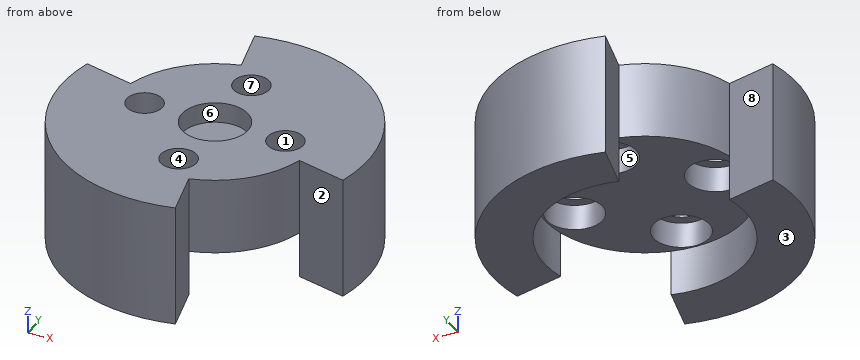
```python
from build123d import *

# Parameters (mm, degrees)
SKETCH012_R     = 9.9
SKETCH012_R_2   = 1.75
PAD009_DEPTH    = 5
SKETCH013_R     = 9.9
SKETCH013_R_2   = 2.75
PAD010_DEPTH    = 2.5
SKETCH014_R     = 3.25
POCKET002_DEPTH = 2
PAD011_DEPTH    = 12


with BuildPart() as part:
    # Sketch012 (on DatumPlane) → Pad009 (new body)
    with BuildSketch(Plane(origin=(0, 0, -19.5), x_dir=(-1, 0, 0), z_dir=(0, 0, -1))):
        Circle(SKETCH012_R)
        with Locations((0, 7)):
            Circle(SKETCH012_R_2, mode=Mode.SUBTRACT)
        with Locations((7, 0)):
            Circle(SKETCH012_R_2, mode=Mode.SUBTRACT)
        with Locations((0, -7)):
            Circle(SKETCH012_R_2, mode=Mode.SUBTRACT)
        with Locations((-7, 0)):
            Circle(SKETCH012_R_2, mode=Mode.SUBTRACT)
    extrude(amount=PAD009_DEPTH)

    # Sketch013 (on Face7 of Pad009) → Pad010 (join)
    with BuildSketch(Plane(origin=(0, 0, -24.5), x_dir=(-1, 0, 0), z_dir=(0, 0, -1))):
        Circle(SKETCH013_R)
        with Locations((0, 7)):
            Circle(SKETCH013_R_2, mode=Mode.SUBTRACT)
        with Locations((7, 0)):
            Circle(SKETCH013_R_2, mode=Mode.SUBTRACT)
        with Locations((0, -7)):
            Circle(SKETCH013_R_2, mode=Mode.SUBTRACT)
        with Locations((-7, 0)):
            Circle(SKETCH013_R_2, mode=Mode.SUBTRACT)
    extrude(amount=PAD010_DEPTH)

    # Sketch014 (on DatumPlane) → Pocket002 (cut)
    with BuildSketch(Plane(origin=(0, 0, -19.5), x_dir=(-1, 0, 0), z_dir=(0, 0, -1))):
        Circle(SKETCH014_R)
    extrude(amount=POCKET002_DEPTH, mode=Mode.SUBTRACT)

    # Sketch015 (on DatumPlane) → Pad011 (join)
    with BuildSketch(Plane(origin=(0, 0, -19.5), x_dir=(-1, 0, 0), z_dir=(0, 0, -1))):
        with BuildLine():
            ThreePointArc((2.3686, 9.612478), (-7.000357, 7.000357), (-9.612478, -2.3686))
            Line((-9.612478, -2.3686), (-14.56436, -3.588789))
            ThreePointArc((3.588789, 14.56436), (-10.606602, 10.606602), (-14.56436, -3.588789))
            Line((2.3686, 9.612478), (3.588789, 14.56436))
        make_face()
        with BuildLine():
            Line((9.612478, 2.3686), (14.56436, 3.588789))
            ThreePointArc((-3.588789, -14.56436), (10.606602, -10.606602), (14.56436, 3.588789))
            Line((-2.3686, -9.612478), (-3.588789, -14.56436))
            ThreePointArc((-2.3686, -9.612478), (7.000357, -7.000357), (9.612478, 2.3686))
        make_face()
    extrude(amount=PAD011_DEPTH)


solid = part.part
```
Geometry check sheet. Reference: the model listing, model coordinates, mm. Face numbers are marked on the shaded views. A direction names the side the tool comes from. Coordinates: 2 decimals unless noted, no trailing zeros. Write each loop counter-clockwise with the first axis right and the second up, starting at its lowest first coordinate (ties: lowest second). Pieces come first, ordered by that corner, then holes. Notation, with made-up numbers: (16.5, 88) -> (53.5, 88) arc R15 cw to (53.5, 98) -> close; hole circle Ø5 at (-7.5, -4). An arc over 180 degrees is marked (long way). Use CSV: the item, a comma, the result in double quotes. Start each with the question number.
Item 1: Depth check by flat-ended pin: pin 1 Ø4 at (x, z) = (11.5, -27.5) entering from +Y; pin 2 Ø2 at (y, z) = (-8.5, -24.5) entering from +X; pin 3 Ø1 at (x, z) = (9.5, -26.5) entering from -Y. Enter the tip coordinate at first touch or a pass-through.
Item 2: Cross-section at B-B, the plane y = 7. Record the cut outline in (x, z), plus the area to 3 significant figures.
Item 3: Set-up check for the marked faces 5, 6, 7 and 8: record each of +Z, -Z, +X, -X, +Y, -Y from which the full face is reachable in a straight line by a thin tool's end or side.
Item 4: Cross-section at A-A, the plane x = -1. Record the cut outline in (y, z).
Item 5: Mould release check, pull along Y, two halves, no side actions. Record for the marked faces 1, 2, 3 and 4: released by +Y, released by -Y, zero draft, split by the parting line, or undercut.
Item 6: Thickness scan on line 1 (Y direction, x = 0, z = -25.75); line 2 (Y direction, x = 0, z = -22.85); line 3 (Z direction, x = 5.5, y = 4.75). Record the ranges inside material, lowest first.
Item 7: Cross-section at C-C, the plane z = -25.75. Record the cut outline in (x, y).
Answers:
1,pin 1,"y = 11.61"
1,pin 2,"x = 6.46"
1,pin 3,"y = -4.12"
2,outline,"(-7, -27) -> (-2.75, -27) -> (-2.75, -24.5) -> (-1.75, -24.5) -> (-1.75, -19.5) -> (-7, -19.5) -> close; (1.75, -24.5) -> (2.75, -24.5) -> (2.75, -27) -> (7, -27) -> (7, -31.5) -> (13.27, -31.5) -> (13.27, -19.5) -> (1.75, -19.5) -> close"
2,area,"149 mm^2"
3,face 5,"-Z"
3,face 6,"+Z"
3,face 7,"+Z, -Z"
3,face 8,"+Z, -Z, +Y"
4,outline,"(-14.97, -31.5) -> (-9.85, -31.5) -> (-9.85, -27) -> (-9.56, -27) -> (-9.56, -24.5) -> (-8.44, -24.5) -> (-8.44, -19.5) -> (-14.97, -19.5) -> close; (-5.56, -24.5) -> (-4.44, -24.5) -> (-4.44, -27) -> (4.44, -27) -> (4.44, -24.5) -> (5.56, -24.5) -> (5.56, -19.5) -> (3.09, -19.5) -> (3.09, -21.5) -> (-3.09, -21.5) -> (-3.09, -19.5) -> (-5.56, -19.5) -> close; (8.44, -24.5) -> (9.56, -24.5) -> (9.56, -27) -> (9.85, -27) -> (9.85, -31.5) -> (14.97, -31.5) -> (14.97, -19.5) -> (8.44, -19.5) -> close"
5,face 1,"undercut"
5,face 2,"released by -Y"
5,face 3,"zero draft"
5,face 4,"undercut"
6,line 1,"-15 to -9.75, -4.25 to 4.25, 9.75 to 15"
6,line 2,"-15 to -8.75, -5.25 to 5.25, 8.75 to 15"
6,line 3,"-27 to -19.5"
7,outline,"(-14.56, 3.59) arc R15 ccw to (3.59, -14.56) -> (2.37, -9.61) arc R9.9 ccw to (9.61, -2.37) -> (14.56, -3.59) arc R15 ccw to (-3.59, 14.56) -> (-2.37, 9.61) arc R9.9 ccw to (-9.61, 2.37) -> close; hole circle Ø5.5 at (-7, 0); hole circle Ø5.5 at (0, -7); hole circle Ø5.5 at (0, 7); hole circle Ø5.5 at (7, 0)"
